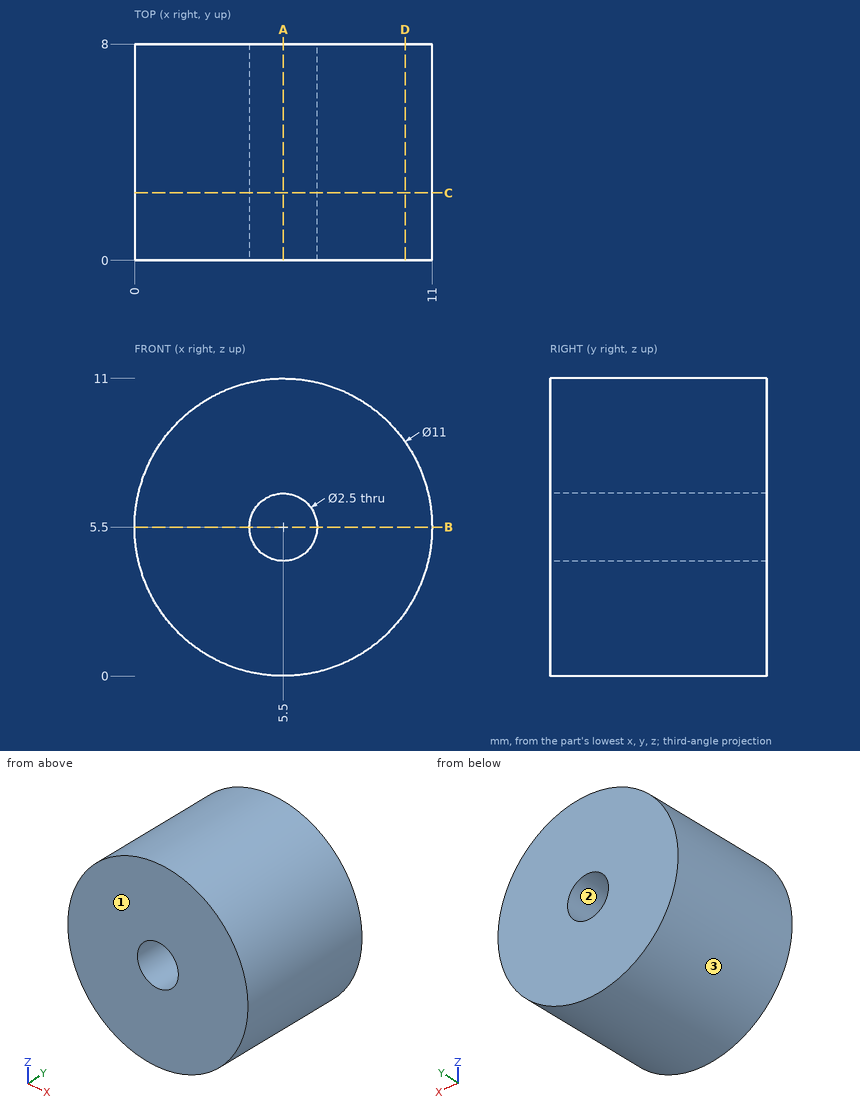
Geometry: see drawing. Coordinates: mm, zero at the bounding-box minimum. Coordinates: 2 decimals unless noted, no trailing zeros. Loops run counter-clockwise (first coordinate to the right, second up) from the corner with the lowest first, then second, coordinate; pieces in that order, holes last. Notation, with made-up numbers: (-2, 3) -> (26, 3) arc R16 ccw to (26, 26) -> close; hole circle Ø9 at (-30, 19). An arc over 180 degrees is marked (long way). Write item = value, one per line. Start each with the question number.
Item 1: Cut plane D-D, the plane x = 10. Return loops of the section in (y, z), plus the area to 3 significant figures.
Item 2: Material intervals for line 1 (Z direction, x = 5.5, y = 4); line 2 (Z direction, x = 4.75, y = 2.75), sorted ascending.
Item 3: Cut plane B-B, the plane z = 5.5. Return loops of the section in (x, y).
Item 4: Cut plane A-A, the plane x = 5.5. Return loops of the section in (y, z), plus the area to 3 significant figures.
Item 5: First-contact query: P1, Ø1, axis at x = 2, y = 4, coming from the -Z side; P2, Ø4, axis at y = 6, z = 8.5, coming from the +X side; P3, Ø3, axis at y = 4.5, z = 3, coming from the -X side. Flat tips, straight axial feed; report the tip coordinate or a pass-through.
Item 6: Cut plane C-C, the plane y = 2.5. Return loops of the section in (x, z).
Item 7: Mould query, pull axis Z, two halves, no side actions, for the marked faces 1, 2 and 3. Classes: pulls with the +Z half, pulls with the -Z half, needs draft (parallel to the pull), parting line crosses it, or undercut.
Ans:
q1.outline = (0, 2.34) -> (8, 2.34) -> (8, 8.66) -> (0, 8.66) -> close
q1.area = 50.6 mm²
q2.line_1 = 0 to 4.25, 6.75 to 11
q2.line_2 = 0.05 to 4.5, 6.5 to 10.95
q3.outline = (0, 0) -> (4.25, 0) -> (4.25, 8) -> (0, 8) -> close; (6.75, 0) -> (11, 0) -> (11, 8) -> (6.75, 8) -> close
q4.outline = (0, 0) -> (8, 0) -> (8, 4.25) -> (0, 4.25) -> close; (0, 6.75) -> (8, 6.75) -> (8, 11) -> (0, 11) -> close
q4.area = 68.0 mm²
q5.P1 = 0.89
q5.P2 = 10.91
q5.P3 = 0.09
q6.outline = circle Ø11 at (5.5, 5.5); hole circle Ø2.5 at (5.5, 5.5)
q7.face_1 = needs draft
q7.face_2 = undercut
q7.face_3 = parting line crosses it
